Work out the finished part from the listing and answer in its coordinate system (mm). A direction names the side the tool comes from. Give positions to 0.01 mm unless a question says otherwise; leave off trailing zeros. Write each loop counter-clockwise with the first axis right and the second up, starting at its lowest first coordinate (ties: lowest second). Pieces come first, ordered by that corner, then holes.
1) Determine the mould class of faces 4 (the face through (1, -36, 9.525)), 5 (the face through (39.464, 61.59, 0.133)), 6 (the face through (22.225, -17, 18)), 7 (the face through (44.76, -0.36, 37.08)) for opening direction X: pulls with the +X half, pulls with the -X half, needs draft (parallel to the pull), parting line crosses it, or undercut.
2) A tool of negligible diameter and unlimited length cuts with its end or side. For faces 1 (the face through (7, 7.938, 32)), 2 (the face through (61, 2, 42.875)), 3 (the face through (41.275, -1, 4)), from which of +Z, -Z, +X, -X, +Y, -Y can it reach the whole face along a straight path? Write none if from no direction.
3) Straight lines are drawn through the part: probe 1 along Z at (x, y) = (-9, -31.5) (3 decimals); probe 2 along Y at (x, z) = (26.5, 32.5); probe 3 along X at (y, z) = (47, 9) (3 decimals). For each, find the intervals that lie inside material, in ascending order.
4) Given pin 1 Ø0.7 at (y, z) = (2, 62.5) entering from +X; pin 2 Ø8.5 at (y, z) = (15.5, 16.5) entering from -X (3 decimals); pin 3 Ø14 at (x, y) = (69.5, -4.5) entering from -Z, each flat-ended and moving along its own axis, determine where each tip first touches the part or whether it passes through.
5) Find section D-D (x = 95.5). Determine the outline of the cut face in (y, z) (3 decimals).
6) Find section C-C (y = -47.5). Determine the outline of the cut face in (x, z) (3 decimals).
7) Find section A-A (x = 66). Determine the outline of the cut face in (y, z) (3 decimals).
```python
from build123d import *

# Parameters (mm, degrees)
F1_DEPTH = 63.5
F2_DEPTH = 25.4
F3_DEPTH = 7.9375
F4_DEPTH = 25.4
F6_R     = 6.35


with BuildPart() as f1:
    # F0 (on Front) → F1 (new body, symmetric)
    with BuildSketch(Plane.XZ):
        Polygon((-41.275, 9.525), (-41.275, -9.525), (41.275, -9.525), (41.275, 9.525), (22.225, 9.525), align=None)
    extrude(amount=F1_DEPTH, both=True)

    # F0 (on Front) → F2 (join, symmetric)
    with BuildSketch(Plane.XZ):
        with BuildLine():
            Line((22.225, 9.525), (41.275, 9.525))
            Line((41.275, 9.525), (41.275, 27.156549))
            ThreePointArc((41.275, 27.156549), (44.853278, 37.196781), (53.975, 42.710809))
            Line((53.975, 42.710809), (53.975, 61.936932))
            ThreePointArc((53.975, 61.936932), (31.356178, 50.70298), (22.225, 27.156549))
            Line((22.225, 27.156549), (22.225, 9.525))
        make_face()
    extrude(amount=F2_DEPTH, both=True)

    # F0 (on Front) → F3 (join, symmetric)
    with BuildSketch(Plane.XZ):
        with BuildLine():
            add(Edge.make_bspline(
                [(-41.275, 9.525), (-28.28964, 37.114333), (17.647352, 65.702192), (53.975, 62.803717)],
                knots=[0, 0, 0, 0, 107.903289, 107.903289, 107.903289, 107.903289], degree=3))
            Line((-41.275, 9.525), (22.225, 9.525))
            Line((22.225, 9.525), (22.225, 27.156549))
            ThreePointArc((22.225, 27.156549), (31.356178, 50.70298), (53.975, 61.936932))
            Line((53.975, 61.936932), (53.975, 62.803717))
        make_face()
    extrude(amount=F3_DEPTH, both=True)

    # F0 (on Front) → F4 (join, symmetric)
    with BuildSketch(Plane.XZ):
        with BuildLine():
            ThreePointArc((60.450994, 61.9252), (57.21327, 62.081492), (53.975, 61.936932))
            Line((53.975, 61.936932), (53.975, 42.710809))
            ThreePointArc((53.975, 42.710809), (56.666725, 43.024192), (59.372532, 42.8752))
            Line((59.372532, 42.8752), (89.295853, 42.8752))
            Line((89.295853, 42.8752), (89.295853, 61.9252))
            Line((89.295853, 61.9252), (60.450994, 61.9252))
        make_face()
    extrude(amount=F4_DEPTH, both=True)

    # F0 (on Front) → F5 (revolve)
    with BuildSketch(Plane.XZ):
        Polygon((117.475, 66.675), (89.295853, 66.675), (89.295853, 61.9252), (89.295853, 42.8752), (89.295853, 38.1), (117.475, 38.1), align=None)
    revolve(axis=Axis((89.295853, 0, 52.3875), (0, 0, 1)))

    # F6
    f6_edges = [f1.edges().sort_by_distance(p)[0] for p in [
        (41.275, -63.5, 0),
        (-41.275, -63.5, 0),
        (-41.275, 63.5, 0),
        (41.275, 63.5, 0),
    ]]
    fillet(f6_edges, radius=F6_R)


solid = f1.part
```
Results:
1. face 4: needs draft
1. face 5: pulls with the +X half
1. face 6: pulls with the -X half
1. face 7: undercut
2. face 1: +Z, -X, +Y
2. face 2: -Z
2. face 3: -Z, +X, +Y, -Y
3. probe 1: z = -9.525 to 9.525
3. probe 2: y = -25.4 to 25.4
3. probe 3: x = -41.275 to 41.275
4. pin 1: stops at x = 117.43
4. pin 2: stops at x = 22.225
4. pin 3: stops at z = 38.1
5. outline: (-27.488, 38.1) - (27.488, 38.1) - (27.488, 66.675) - (-27.488, 66.675) - close
6. outline: (-41.275, -9.525) - (41.275, -9.525) - (41.275, 9.525) - (-41.275, 9.525) - close
7. outline: (-25.4, 42.875) - (-15.855, 42.875) - (-15.855, 38.1) - (15.855, 38.1) - (15.855, 42.875) - (25.4, 42.875) - (25.4, 61.925) - (15.855, 61.925) - (15.855, 66.675) - (-15.855, 66.675) - (-15.855, 61.925) - (-25.4, 61.925) - close
